CAD build for the part. Positions are in the model's coordinates, mm. Face numbers are marked on the shaded views. A direction names the side the tool comes from. Coordinates: 2 decimals unless noted, no trailing zeros. Loops run counter-clockwise (first coordinate to the right, second up) from the corner with the lowest first, then second, coordinate; pieces in that order, holes last. Notation, with made-up numbers: (38, 8) -> (93, 8) arc R17 ccw to (93, 36) -> close; hole circle Ø6 at (63.25, 12.5). An arc over 180 degrees is marked (long way). Write each question's results on one line, items separated by ' | '.
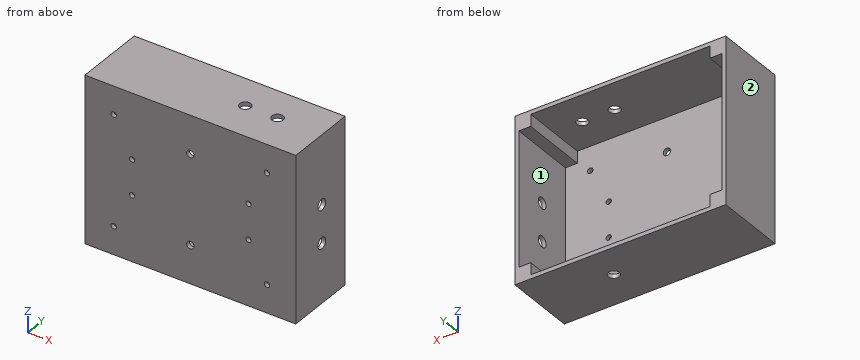
Autodesk Inventor part; units mm, degrees
ref_plane "YZ Plane" through (0, 0, 0) normal (1, 0, 0) x (0, 1, 0)
ref_plane "XZ Plane" through (0, 0, 0) normal (0, 1, 0) x (-1, 0, 0)
ref_plane "XY Plane" through (0, 0, 0) normal (0, 0, 1) x (1, 0, 0)
sketch "Sketch1" plane through (0, 0, 0) normal (0, 1, 0) x (-1, 0, 0)
  line L0 (-59.7535, -47.0027) -> (59.7535, -47.0027)
  line L1 (59.7535, -47.0027) -> (59.7535, 47.0027)
  line L2 (59.7535, 47.0027) -> (-59.7535, 47.0027)
  line L3 (-59.7535, 47.0027) -> (-59.7535, -47.0027)
  line L4 (-59.7535, -47.0027) -> (59.7535, 47.0027) construction
  line L5 (59.7535, -47.0027) -> (-59.7535, 47.0027) construction
  point P0 (0, 0)
  dimension "d0" = 119.507
  dimension "d1" = 94.0054
extrude "Extrusion1" add sketch "Sketch1" along normal mid plane 2.2606
sketch "Sketch2" plane through (0, 1.1303, 0) normal (0, 1, 0) x (1, 0, 0)
  line L0 (-59.7535, 47.0027) -> (-59.7535, -47.0027)
  line L1 (59.7535, -47.0027) -> (59.7535, 47.0027)
  line L2 (-59.7535, -47.0027) -> (59.7535, -47.0027)
  line L3 (59.7535, -47.0027) -> (59.7535, 47.0027)
  line L4 (59.7535, 47.0027) -> (-59.7535, 47.0027)
  line L5 (-59.7535, 47.0027) -> (-59.7535, -47.0027)
  line L6 (57.4929, -44.7421) -> (-57.4929, 44.7421) construction
  line L7 (-57.4929, -44.7421) -> (57.4929, 44.7421) construction
  line L8 (-59.7535, -47.0027) -> (59.7535, -47.0027)
  line L9 (-59.7535, -47.0027) -> (-50.7619, -47.0027)
  line L10 (-59.7535, -38.0111) -> (-59.7535, -47.0027)
  line L11 (-59.7535, 47.0027) -> (-50.7619, 47.0027)
  line L12 (-59.7535, 38.0111) -> (-59.7535, 47.0027)
  line L13 (59.7535, 47.0027) -> (-59.7535, 47.0027)
  line L14 (59.7535, 47.0027) -> (50.7619, 47.0027)
  line L15 (59.7535, 38.0111) -> (59.7535, 47.0027)
  line L16 (59.7535, -47.0027) -> (50.7619, -47.0027)
  line L17 (59.7535, -38.0111) -> (59.7535, -47.0027)
  line L18 (-50.7619, -44.7421) -> (-50.7619, -38.0111)
  line L19 (-50.7619, -38.0111) -> (-57.4929, -38.0111)
  line L20 (-57.4929, 38.0111) -> (-50.7619, 38.0111)
  line L21 (-50.7619, 38.0111) -> (-50.7619, 44.7421)
  line L22 (50.7619, 38.0111) -> (57.4929, 38.0111)
  line L23 (50.7619, 44.7421) -> (50.7619, 38.0111)
  line L24 (57.4929, -38.0111) -> (50.7619, -38.0111)
  line L25 (50.7619, -38.0111) -> (50.7619, -44.7421)
  line L26 (-50.7619, -44.7421) -> (50.7619, -44.7421)
  line L27 (57.4929, -38.0111) -> (57.4929, 38.0111)
  line L28 (50.7619, 44.7421) -> (-50.7619, 44.7421)
  line L29 (-57.4929, 38.0111) -> (-57.4929, -38.0111)
  point P0 (0, 0)
  dimension "d4" = 114.9858
  dimension "d5" = 89.4842
  dimension "d6" = 8.9916
  dimension "d7" = 8.9916
  dimension "d10" = 8.9916
  dimension "d11" = 8.9916
extrude "Extrusion2" add sketch "Sketch2" along normal blind 38.1
sketch "Sketch3" plane through (0, 1.1303, 0) normal (0, 1, 0) x (1, 0, 0)
  circle A0 centre (0, -25.4) radius 2.0828
  circle A1 centre (0, 25.4) radius 2.0828
  point P0 (0, 0)
  dimension "d18" = 4.1656
  dimension "d19" = 4.1656
extrude "Extrusion3" cut sketch "Sketch3" against normal through all
sketch "Sketch7" plane through (0, 1.1303, 0) normal (0, 1, 0) x (1, 0, 0)
  line L0 (44.9961, -32.4993) -> (-44.9961, 32.4993) construction
  line L1 (-44.9961, -32.4993) -> (44.9961, 32.4993) construction
  line L2 (-44.9961, -32.4993) -> (-38.6461, -32.4993) construction
  line L3 (44.9961, -32.4993) -> (64.0461, -32.4993) construction
  line L4 (32.9946, -9.9949) -> (-32.9946, 9.9949) construction
  line L5 (-32.9946, -9.9949) -> (32.9946, 9.9949) construction
  circle A0 centre (-32.9946, -9.9949) radius 1.4986
  circle A1 centre (-32.9946, 9.9949) radius 1.4986
  circle A2 centre (32.9946, -9.9949) radius 1.4986
  circle A3 centre (32.9946, 9.9949) radius 1.4986
  line L6 (-44.45, -32.1469) -> (44.45, -32.1469)
  line L7 (44.45, 32.1469) -> (-44.45, 32.1469)
  line L8 (-44.45, 32.1469) -> (-44.45, -32.1469)
  line L9 (-44.45, -32.1469) -> (44.45, 32.1469) construction
  line L10 (44.45, -32.1469) -> (-44.45, 32.1469) construction
  line L11 (-44.45, -32.1469) -> (-43.434, -32.1469)
  line L12 (-44.45, -31.1309) -> (-44.45, -32.1469)
  circle A4 centre (-43.434, -31.1309) radius 1.524
  line L13 (-44.45, 32.1469) -> (-43.434, 32.1469)
  line L14 (-44.45, 31.1309) -> (-44.45, 32.1469)
  circle A5 centre (-43.434, 31.1309) radius 1.524
  line L15 (44.45, 32.1469) -> (43.434, 32.1469)
  line L16 (44.45, 31.1309) -> (44.45, 32.1469)
  circle A6 centre (43.434, 31.1309) radius 1.524
  line L17 (44.45, -32.1469) -> (43.434, -32.1469)
  line L18 (43.434, -31.1309) -> (44.45, -31.1309)
  circle A7 centre (43.434, -31.1309) radius 1.524
  point P0 (0, 0)
  dimension "d47" = 89.9922
  dimension "d48" = 64.9986
  dimension "d62" = 65.9892
  dimension "d63" = 19.9898
  dimension "d64" = 2.9972
  dimension "d65" = 2.9972
  dimension "d66" = 2.9972
  dimension "d67" = 2.9972
  dimension "d120" = 88.9
  dimension "d121" = 64.2938
  dimension "d124" = 3.048
  dimension "d127" = 3.048
  dimension "d130" = 3.048
  dimension "d131" = 1.016
  dimension "d132" = 1.016
  dimension "d133" = 3.048
sketch "Sketch8" plane through (-50.7619, 1.1303, -44.7421) normal (0, 0, 1) x (1, 0, 0)
  line L0 (0, 0) -> (0, 38.1)
  circle A0 centre (67.6783, 19.05) radius 3.175
  point P0 (50.7619, -1.1303)
  dimension "d99" = 6.35
extrude "Extrusion7" cut sketch "Sketch8" against normal through all
sketch "Sketch10" plane through (57.4929, 1.1303, -38.0111) normal (-1, 0, 0) x (0, 0, 1)
  line L0 (0, 0) -> (0, 38.1)
  line L1 (0, 19.05) -> (5.5118, 19.05) construction
  circle A0 centre (24.5618, 19.05) radius 3.175
  circle A1 centre (45.993, 19.05) radius 3.175
  point P0 (38.0111, -1.1303)
  dimension "d118" = 6.35
  dimension "d119" = 6.35
extrude "Extrusion8" cut sketch "Sketch10" against normal through all
sketch "Sketch11" plane through (50.7619, 1.1303, 44.7421) normal (0, 0, -1) x (-1, 0, 0)
  line L0 (101.5238, 0) -> (101.5238, 38.1)
  line L1 (101.5238, 19.05) -> (95.758, 19.05)
  line L2 (0, 0) -> (0, 38.1)
  line L3 (0, 0) -> (0, 38.1)
  circle A0 centre (16.0846, 19.05) radius 3.175
  circle A1 centre (34.3408, 19.05) radius 3.175
  point P0 (50.7619, -1.1303)
  dimension "d80" = 5.7658
  dimension "d112" = 6.35
  dimension "d113" = 6.35
extrude "Extrusion9" cut sketch "Sketch11" against normal through all
extrude "Extrusion10" cut sketch "Sketch7" against normal through all
properties part number "546-1590BBS-ADF41020"
Q1. Cut at A-A on z = 25.4. Write the cut outline in (x, y).
Results are:
outline: (-59.75, -1.13) -> (-2.08, -1.13) -> (-2.08, 1.13) -> (-57.49, 1.13) -> (-57.49, 39.23) -> (-59.75, 39.23) -> close; (2.08, -1.13) -> (59.75, -1.13) -> (59.75, 39.23) -> (57.49, 39.23) -> (57.49, 1.13) -> (2.08, 1.13) -> close
Q2. Cut at B-B on y = 10.5. Write the cut outline in (x, z).
Results are:
outline: (-59.75, -47) -> (59.75, -47) -> (59.75, 47) -> (-59.75, 47) -> close; hole (-57.49, -38.01) -> (-50.76, -38.01) -> (-50.76, -44.74) -> (50.76, -44.74) -> (50.76, -38.01) -> (57.49, -38.01) -> (57.49, 38.01) -> (50.76, 38.01) -> (50.76, 44.74) -> (-50.76, 44.74) -> (-50.76, 38.01) -> (-57.49, 38.01) -> close
Q3. Wall check: L1, parallel to Z at x = 0, y = 0; L2, parallel to X at y = 28, z = 39; L3, parallel to X at y = 24, z = 31.5. Give the ranges that are in metal, low to high. Write a range as from..to.
Results are:
L1: -47..-27.48, -23.32..23.32, 27.48..47 | L2: -59.75..-50.76, 50.76..59.75 | L3: -59.75..-57.49, 57.49..59.75
Q4. Cut at C-C on x = -23. Write the cut outline in (y, z), and give its area (3 significant figures).
Results are:
outline: (-1.13, -47) -> (39.23, -47) -> (39.23, -44.74) -> (1.13, -44.74) -> (1.13, 44.74) -> (39.23, 44.74) -> (39.23, 47) -> (-1.13, 47) -> close | area: 385 mm^2
Q5. Drop a flat-ended pin along its axis: pin 1 (4 mm diameter, centred on x = 32.99, z = -9.99, fed in from +Y). Give the stop position or say it passes through.
Results are:
pin 1: y = 1.13
Q6. Cut at D-D on z = 1. Write the cut outline in (x, y), and give its area (3 significant figures).
Results are:
outline: (-59.75, -1.13) -> (59.75, -1.13) -> (59.75, 39.23) -> (57.49, 39.23) -> (57.49, 1.13) -> (-57.49, 1.13) -> (-57.49, 39.23) -> (-59.75, 39.23) -> close | area: 442 mm^2
Q7. Which spindle directions (+Z, -Z, +X, -X, +Y, -Y) get a long thin tool onto all of the face, cutting with end or side? Do the marked faces 1 and 2. Say none if no direction does.
Results are:
face 1: +Y | face 2: +Z, -Z, -X, +Y, -Y
